```python
from build123d import *
from build123d.topology import SkipClean

# Parameters (mm, degrees)
SKETCH1_W                                       = 300
SKETCH1_H                                       = 100
BOSS_EXTRUDE1_DEPTH                             = 20
CSK_FOR_M2_FLAT_HEAD_MACHINE_SCREW1_D           = 2.4
CSK_FOR_M2_FLAT_HEAD_MACHINE_SCREW1_DEPTH       = 15
CSK_FOR_M2_FLAT_HEAD_MACHINE_SCREW1_CSINK_D     = 4.4
CSK_FOR_M2_FLAT_HEAD_MACHINE_SCREW1_CSINK_ANGLE = 90
CSK_FOR_M2_FLAT_HEAD_MACHINE_SCREW1_TIP         = 0.721032743
SKETCH5_W                                       = 40
SKETCH5_H                                       = 20
CUT_EXTRUDE1_DEPTH                              = 160.373774505
SHELL1_START                                    = 1.4
SHELL1_OUTLINE_W                                = 297.2
SHELL1_OUTLINE_H                                = 97.2
SHELL1_OUTLINE_R                                = 2.6
SHELL1_OUTLINE_W_2                              = 42.8
SHELL1_OUTLINE_H_2                              = 22.8
SHELL1_DEPTH                                    = 17.020100913
SHELL1_2_OUTLINE_R                              = 2.6
SHELL1_2_DEPTH                                  = 1.245680401
SHELL1_START_2                                  = 18.420101013
SHELL1_4_OUTLINE_W                              = 297.2
SHELL1_4_OUTLINE_H                              = 97.2
SHELL1_4_OUTLINE_W_2                            = 42.8
SHELL1_4_OUTLINE_H_2                            = 22.8
SHELL1_4_OUTLINE_W_3                            = 40
SHELL1_4_OUTLINE_H_3                            = 20
SHELL1_4_DEPTH                                  = 0.179898987
CBORE_FOR_M5_HEX_HEAD_BOLT1_D                   = 5.5
CBORE_FOR_M5_HEX_HEAD_BOLT1_CBORE_D             = 12.24
CBORE_FOR_M5_HEX_HEAD_BOLT1_CBORE_DEPTH         = 3.58


with BuildPart() as part:
    # Sketch1 → Boss-Extrude1 (new body)
    with BuildSketch(Plane(origin=(0, 0, 0), x_dir=(1, 0, 0), z_dir=(0, 1, 0))):
        Rectangle(SKETCH1_W, SKETCH1_H)
    extrude(amount=BOSS_EXTRUDE1_DEPTH)

    # CSK for M2 Flat Head Machine Screw1
    with Locations(Plane(origin=(0, 20, 0), x_dir=(1, 0, 0), z_dir=(0, 1, 0))):
        with Locations((-120, 0), (-106, 0), (-113.505077549, 6.60861642), (-113.505077549, -7.39138358)):
            CounterSinkHole(CSK_FOR_M2_FLAT_HEAD_MACHINE_SCREW1_D / 2, CSK_FOR_M2_FLAT_HEAD_MACHINE_SCREW1_CSINK_D / 2, depth=CSK_FOR_M2_FLAT_HEAD_MACHINE_SCREW1_DEPTH, counter_sink_angle=CSK_FOR_M2_FLAT_HEAD_MACHINE_SCREW1_CSINK_ANGLE)
            with Locations((0, 0, -(CSK_FOR_M2_FLAT_HEAD_MACHINE_SCREW1_DEPTH + CSK_FOR_M2_FLAT_HEAD_MACHINE_SCREW1_TIP / 2))):  # 118° drill point
                Cone(0, CSK_FOR_M2_FLAT_HEAD_MACHINE_SCREW1_D / 2, CSK_FOR_M2_FLAT_HEAD_MACHINE_SCREW1_TIP, mode=Mode.SUBTRACT)

    # Sketch5 → Cut-Extrude1 (cut, through all)
    with BuildSketch(Plane(origin=(0, 20, 0), x_dir=(1, 0, 0), z_dir=(0, 1, 0))):
        with Locations((100, 0)):
            Rectangle(SKETCH5_W, SKETCH5_H)
    extrude(amount=-CUT_EXTRUDE1_DEPTH, mode=Mode.SUBTRACT)

    # Shell1: read off the stored shape, not the designer's step
    # Shell1 outline → Shell1 (cut)
    with BuildSketch(Plane(origin=(0, 0, 0), x_dir=(1, 0, 0), z_dir=(0, 1, 0)).offset(SHELL1_START)):
        Rectangle(SHELL1_OUTLINE_W, SHELL1_OUTLINE_H)
        with Locations((-113.505077549, -7.39138358)):
            Circle(SHELL1_OUTLINE_R, mode=Mode.SUBTRACT)
        with Locations((-120, 0)):
            Circle(SHELL1_OUTLINE_R, mode=Mode.SUBTRACT)
        with Locations((-113.505077549, 6.60861642)):
            Circle(SHELL1_OUTLINE_R, mode=Mode.SUBTRACT)
        with Locations((-106, 0)):
            Circle(SHELL1_OUTLINE_R, mode=Mode.SUBTRACT)
        with Locations((100, 0)):
            Rectangle(SHELL1_OUTLINE_W_2, SHELL1_OUTLINE_H_2, mode=Mode.SUBTRACT)
    extrude(amount=SHELL1_DEPTH, mode=Mode.SUBTRACT)

    # Shell1 2 outline → Shell1 2 (cut)
    with BuildSketch(Plane(origin=(0, 0, 0), x_dir=(1, 0, 0), z_dir=(0, 1, 0)).offset(SHELL1_START)):
        with Locations((-113.505077549, -7.39138358)):
            Circle(SHELL1_2_OUTLINE_R)
        with Locations((-113.505077549, 6.60861642)):
            Circle(SHELL1_2_OUTLINE_R)
        with Locations((-106, 0)):
            Circle(SHELL1_2_OUTLINE_R)
        with Locations((-120, 0)):
            Circle(SHELL1_2_OUTLINE_R)
    extrude(amount=SHELL1_2_DEPTH, mode=Mode.SUBTRACT)

    # Shell1 3 outline → Shell1 3 (revolve, cut)
    with BuildSketch(Plane(origin=(-113.505077549, 0, 7.39138358), x_dir=(1, 0, 0), z_dir=(0, 0, 1))):
        Polygon((268.018855143, 18.6), (2.779898987, 18.6), (2.6, 18.420101013), (268.018855143, 18.420101013), align=None)
        Polygon((2.6, 2.645680501), (2.6, 4.207918111), (0, 2.645680501), align=None)
    revolve(axis=Axis((-113.505077549, 0, 7.39138358), (0, 1, 0)), mode=Mode.SUBTRACT)

    # Shell1 4 outline → Shell1 4 (add)
    # profile 1 of 2: a face of its own
    with BuildSketch(Plane(origin=(0, 0, 0), x_dir=(1, 0, 0), z_dir=(0, 1, 0)).offset(SHELL1_START_2)):
        with BuildLine():
            Line((150, -50), (150, 41.590049821))
            ThreePointArc((150, 41.590049821), (149.323371513, 45.099692578), (148.6, 48.6))
            ThreePointArc((148.6, 48.6), (148.449442912, 49.300202411), (148.297015267, 50))
            Line((148.297015267, 50), (-150, 50))
            Line((-150, 50), (-150, -50))
            Line((-150, -50), (150, -50))
        make_face()
        Rectangle(SHELL1_4_OUTLINE_W, SHELL1_4_OUTLINE_H, mode=Mode.SUBTRACT)
    # profile 2 of 2: a face of its own
    with BuildSketch(Plane(origin=(0, 0, 0), x_dir=(1, 0, 0), z_dir=(0, 1, 0)).offset(SHELL1_START_2)):
        with Locations((100, 0)):
            Rectangle(SHELL1_4_OUTLINE_W_2, SHELL1_4_OUTLINE_H_2)
        with Locations((100, 0)):
            Rectangle(SHELL1_4_OUTLINE_W_3, SHELL1_4_OUTLINE_H_3, mode=Mode.SUBTRACT)
    extrude(amount=SHELL1_4_DEPTH)

    # Shell1 5 outline → Shell1 5 (revolve)
    with SkipClean():  # the faces are left unmerged after this step: merging them gives an invalid solid
        with BuildSketch(Plane(origin=(-113.505077549, 0, -6.60861642), x_dir=(1, 0, 0), z_dir=(0, 0, 1))):
            Polygon((2.779898987, 18.6), (1.2, 18.6), (1.2, 18.420101013), (2.6, 18.420101013), align=None)
        revolve(axis=Axis((-113.505077549, 0, -6.60861642), (0, 1, 0)))
    add(part.part.scale(1), mode=Mode.REPLACE)  # the faces are merged on a copy

    # Shell1 6 outline → Shell1 6 (revolve)
    with SkipClean():  # the faces are left unmerged after this step: merging them gives an invalid solid
        with BuildSketch(Plane(origin=(-106, 0, 0), x_dir=(1, 0, 0), z_dir=(0, 0, 1))):
            Polygon((2.779898987, 18.6), (1.2, 18.6), (1.2, 18.420101013), (2.6, 18.420101013), align=None)
        revolve(axis=Axis((-106, 0, 0), (0, 1, 0)))
    add(part.part.scale(1), mode=Mode.REPLACE)  # the faces are merged on a copy

    # Shell1 7 outline → Shell1 7 (revolve)
    with SkipClean():  # the faces are left unmerged after this step: merging them gives an invalid solid
        with BuildSketch(Plane(origin=(-120, 0, 0), x_dir=(1, 0, 0), z_dir=(0, 0, 1))):
            Polygon((2.779898987, 18.6), (1.2, 18.6), (1.2, 18.420101013), (2.6, 18.420101013), align=None)
        revolve(axis=Axis((-120, 0, 0), (0, 1, 0)))
    add(part.part.scale(1), mode=Mode.REPLACE)  # the faces are merged on a copy

    # Shell1 8 outline → Shell1 8 (revolve, cut)
    with BuildSketch(Plane(origin=(-113.505077549, 0, -6.60861642), x_dir=(1, 0, 0), z_dir=(0, 0, 1))):
        Polygon((0, 2.645680426), (2.6, 2.645680401), (2.6, 4.207918111), align=None)
    revolve(axis=Axis((-113.505077549, 0, -6.60861642), (0, 1, 0)), mode=Mode.SUBTRACT)

    # Shell1 9 outline → Shell1 9 (revolve, cut)
    with BuildSketch(Plane(origin=(-106, 0, 0), x_dir=(1, 0, 0), z_dir=(0, 0, 1))):
        Polygon((0, 2.645680426), (2.6, 2.645680401), (2.6, 4.207918111), align=None)
    revolve(axis=Axis((-106, 0, 0), (0, 1, 0)), mode=Mode.SUBTRACT)

    # Shell1 10 outline → Shell1 10 (revolve, cut)
    with BuildSketch(Plane(origin=(-120, 0, 0), x_dir=(1, 0, 0), z_dir=(0, 0, 1))):
        Polygon((0, 2.645680426), (2.6, 2.645680401), (2.6, 4.207918111), align=None)
    revolve(axis=Axis((-120, 0, 0), (0, 1, 0)), mode=Mode.SUBTRACT)

    # CBORE for M5 Hex Head Bolt1 (through all)
    with Locations(Plane(origin=(0, 0, -50), x_dir=(-1, 0, 0), z_dir=(0, 0, -1))):
        with Locations((0, 10), (-100, 10), (100, 10)):
            CounterBoreHole(CBORE_FOR_M5_HEX_HEAD_BOLT1_D / 2, CBORE_FOR_M5_HEX_HEAD_BOLT1_CBORE_D / 2, CBORE_FOR_M5_HEX_HEAD_BOLT1_CBORE_DEPTH)


solid = part.part
```
Design review of the part built by this model. Coordinates are the model's own, in mm. A direction names the side the tool comes from. Coordinates: 2 decimals unless noted, no trailing zeros. Write each loop counter-clockwise with the first axis right and the second up, starting at its lowest first coordinate (ties: lowest second). Pieces come first, ordered by that corner, then holes.
1) Add section D-D (y = 10). State how many separate pieces and enclosed holes the cut face has, plus the area to 3 significant figures.
2) Machinability: for faces 1 (the cylindrical face through (94.163, 11.838, -49.31)), 2 (the flat face through (-2, 4, -48.6)), 3 (the flat face through (80, 10, 0)), 4 (the cylindrical face through (97.253, 10.121, 49.31)), 5 (the flat face through (-2, 0, -1)), which of the approach directions +Z, -Z, +X, -X, +Y, -Y give a long, thin tool a straight path to every point of the face, cutting with its end or side? Answer none if there is none.
3) Add section B-B (x = 0). Write out the cut boundary in (y, z), plus the area to 3 significant figures.
4) Add section A-A (z = 38.5). Write out the cut boundary in (x, y), plus the area to 3 significant figures.
5) Add section C-C (x = -61.5). Write out the cut boundary in (y, z).
6) Mouldability with a two-part tool opening along Z and no side actions: class faces 6 (the cylindrical face through (-0.358, 12.727, 49.31)), 7 (the flat face through (95, 10, -10)), 8 (the flat face through (-2.1, 12.1, 50)) as +Z half, -Z half, draft (parallel to the pull), parting line (faces both ways), or undercut.
7) Insertion check: pin 1 (9 mm diameter, centred on x = 100, y = 10, fed in from -Z); pin 2 (10 mm diameter, centred on x = -100, y = 10, fed in from -Z); pin 3 (1.5 mm diameter, centred on x = 100.5, y = 12, fed in from +Z); pin 4 (3 mm diameter, centred on x = -106, z = 0, fed in from +Y). Each pin has a flat end and moves straight along its axis. Give the tip position at first contact, or say it passes through.
8) To check wall thickness, follow L1, parallel to Z at x = 87.5, y = 5; L2, parallel to Z at x = -90, y = 3.75; L3, parallel to X at y = 11, z = 25. State the ranges of each line that lie inside material, in increasing order.
Check result:
1. separate pieces: 12
1. enclosed holes: 4
1. area: 1,260 mm2
2. face 1: -Z
2. face 2: none
2. face 3: +Y, -Y
2. face 4: +Z, -Z
2. face 5: +Z, -Z, +X, -X, -Y
3. outline: (0, -50) - (3.88, -50) - (3.88, -48.6) - (1.4, -48.6) - (1.4, 48.6) - (7.25, 48.6) - (7.25, 50) - (0, 50) - close; (12.75, 48.6) - (18.6, 48.6) - (18.6, -48.6) - (16.12, -48.6) - (16.12, -50) - (20, -50) - (20, 50) - (12.75, 50) - close
3. area: 303 mm2
4. outline: (-150, 0) - (150, 0) - (150, 20) - (-150, 20) - close; hole (-148.6, 1.4) - (148.6, 1.4) - (148.6, 18.6) - (-148.6, 18.6) - close
4. area: 888 mm2
5. outline: (0, -50) - (20, -50) - (20, 50) - (0, 50) - close; hole (1.4, -48.6) - (18.6, -48.6) - (18.6, 48.6) - (1.4, 48.6) - close
6. face 6: draft
6. face 7: undercut
6. face 8: +Z half
7. pin 1: stops at z = -11.4
7. pin 2: stops at z = -2.4
7. pin 3: stops at z = 50
7. pin 4: stops at y = 19.3
8. L1: z = -50 to -48.6, -11.4 to -10, 10 to 11.4, 48.6 to 50
8. L2: z = -50 to -48.6, 48.6 to 50
8. L3: x = -150 to -148.6, 148.6 to 150
